The drawing under review shows one solid part. Ordinate dimensions are in mm from its lowest x, y, z. A direction names the side the tool comes from. Round coordinates to 2 decimals unless told otherwise and drop trailing zeros. Write each loop counter-clockwise with the first axis right and the second up, starting at its lowest first coordinate (ties: lowest second). Pieces come first, ordered by that corner, then holes. Notation, with made-up numbers: (43.25, 42) -> (62.25, 42) arc R27 cw to (62.25, 69) -> close; hole circle Ø1 at (51.25, 55). An arc over 180 degrees is marked (long way). Write item = value, one per line. Start each with the question number.
Item 1: Add section B-B, the plane y = 1. State the section outline as (x, z) points.
Item 2: Machinability: for the marked faces 1 and 2, which of the approach directions +Z, -Z, +X, -X, +Y, -Y give a long, thin tool a straight path to every point of the face, cutting with its end or side? Answer none if there is none.
Item 3: Add section C-C, the plane z = 5.35. State the section outline as (x, y) points (1 decimal).
Item 4: Add section D-D, the plane x = 4.7. State the section outline as (y, z) points.
Item 5: Add section A-A, the plane x = 3. State the section outline as (y, z) points.
Item 6: To check wall thickness, follow L1, parallel to Y at x = 3.25, z = 5.3; L2, parallel to Y at x = 2.35, z = 2.7; L3, parallel to Z at x = 2.25, y = 5. State the ranges of each line that lie inside material, in increasing order.
Item 7: Mouldability with a two-part tool opening along X and no side actions: class the marked faces 3, 4 and 5 as released by +X, released by -X, zero draft, split by the parting line, or undercut.
Item 8: For pin 1 Ø1 at (x, y) = (4, 7) entering from +Z (1 decimal); pin 2 Ø2 at (x, y) = (3.5, 7) entering from -Z; pin 3 Ø1 at (y, z) = (1, 0.5) entering from -X; pin 4 Ø1.8 at (x, z) = (3, 1.5) entering from +Y, all flat-tipped, find the tip position at first contact; note any pin that passes through.
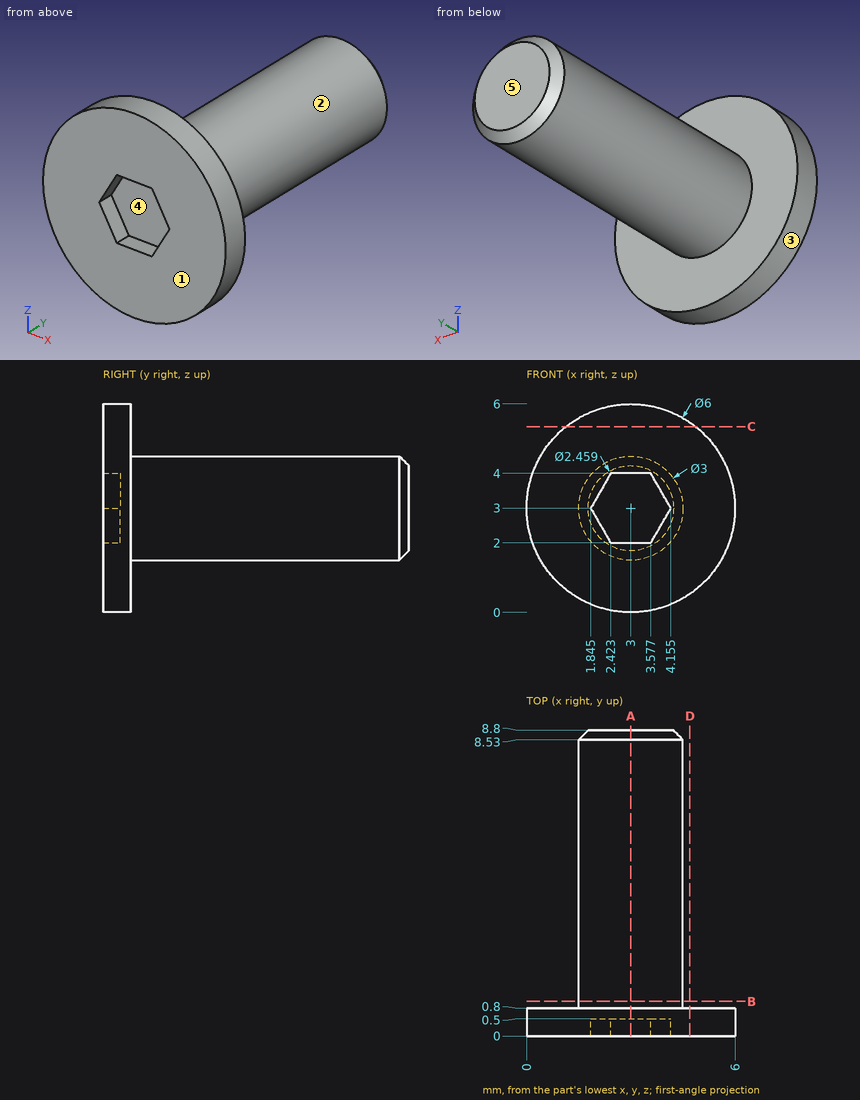
Result set:
q1.outline = circle Ø3 at (3, 3)
q2.face_1 = +Z, -Z, +X, -X, -Y
q2.face_2 = +Y
q3.outline = (1.1, 0) -> (4.9, 0) -> (4.9, 0.8) -> (1.1, 0.8) -> close
q4.outline = (0, 0.53) -> (0.8, 0.53) -> (0.8, 5.47) -> (0, 5.47) -> close
q5.outline = (0, 0) -> (0.8, 0) -> (0.8, 1.5) -> (8.53, 1.5) -> (8.8, 1.77) -> (8.8, 4.23) -> (8.53, 4.5) -> (0.8, 4.5) -> (0.8, 6) -> (0, 6) -> (0, 4) -> (0.5, 4) -> (0.5, 2) -> (0, 2) -> close
q6.L1 = 0 to 0.8
q6.L2 = 0.5 to 8.8
q6.L3 = 1.7 to 4.3
q7.face_3 = split by the parting line
q7.face_4 = undercut
q7.face_5 = zero draft
q8.pin_1 = 4.4
q8.pin_2 = 1.5
q8.pin_3 = 0.8
q8.pin_4 = 8.8
